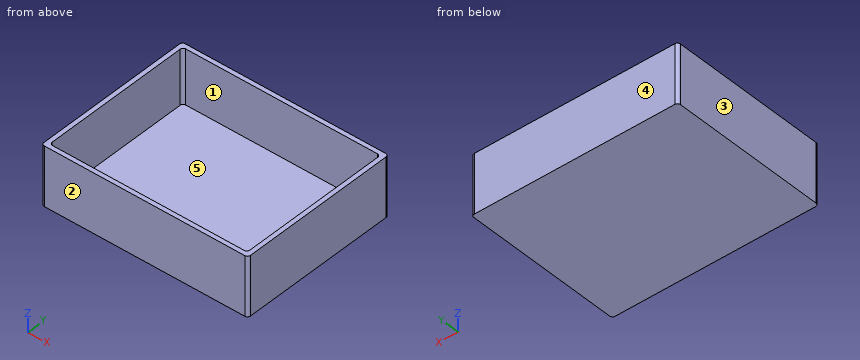
from build123d import *

# Parameters (mm, degrees)
F0_W     = 70
F0_H     = 55
F1_DEPTH = 20
F2_T     = -1.5
F3_R     = 1
F4_R     = 1
F5_R     = 1
F6_R     = 1
F7_R     = 1
F8_R     = 1
F9_R     = 1


with BuildPart() as f1:
    # F0 (on Top) → F1 (new body)
    with BuildSketch(Plane.XY):
        with Locations((35, 27.5)):
            Rectangle(F0_W, F0_H)
    extrude(amount=F1_DEPTH)

    # F2
    f2_openings = [f1.faces().sort_by_distance(p)[0] for p in [
        (35, 27.5, 20),
    ]]
    offset(amount=F2_T, openings=f2_openings)

    # F3
    f3_edges = [f1.edges().sort_by_distance(p)[0] for p in [
        (0, 55, 10),
        (1.5, 53.5, 10.75),
    ]]
    fillet(f3_edges, radius=F3_R)

    # F4
    f4_edges = [f1.edges().sort_by_distance(p)[0] for p in [
        (0, 0, 10),
    ]]
    fillet(f4_edges, radius=F4_R)

    # F5
    f5_edges = [f1.edges().sort_by_distance(p)[0] for p in [
        (70, 0, 10),
    ]]
    fillet(f5_edges, radius=F5_R)

    # F6
    f6_edges = [f1.edges().sort_by_distance(p)[0] for p in [
        (70, 55, 10),
    ]]
    fillet(f6_edges, radius=F6_R)

    # F7
    f7_edges = [f1.edges().sort_by_distance(p)[0] for p in [
        (68.5, 1.5, 10.75),
    ]]
    fillet(f7_edges, radius=F7_R)

    # F8
    f8_edges = [f1.edges().sort_by_distance(p)[0] for p in [
        (1.5, 1.5, 10.75),
    ]]
    fillet(f8_edges, radius=F8_R)

    # F9
    f9_edges = [f1.edges().sort_by_distance(p)[0] for p in [
        (68.5, 53.5, 10.75),
    ]]
    fillet(f9_edges, radius=F9_R)


solid = f1.part
Geometry: final body of the model. Coordinates: model frame, mm. Face numbers are marked on the shaded views. A direction names the side the tool comes from. Round coordinates to 2 decimals unless told otherwise and drop trailing zeros. Order: outer loops, then holes, each group sorted by start corner. A loop starts at its lowest first (then second) coordinate and runs counter-clockwise, first axis right, second up. Notation, with made-up numbers: (61, 26) -> (68, 26) arc R37 ccw to (68, 64) -> close; hole circle Ø2 at (49.25, 29.25). An arc over 180 degrees is marked (long way). Put each result on its own line as item: value. Start each with the question number.
Q1. Pull-direction query (Y, two-part tool) for the marked faces 1, 2 and 3; classes: +Y half, -Y half, draft (parallel to the pull), parting line (faces both ways), or undercut.
Q2. Reachability of the marked faces 4 and 5 from +Z, -Z, +X, -X, +Y, -Y: full face, straight path, thin tool, end or side. Return the list, or none.
Q3. Section A-A on x = 23. Return the cut outline in (y, z), and give its area (3 significant figures).
Q4. Section B-B on y = 6.5. Return the cut outline in (x, z).
Q5. First-contact query: pin 1 (4 mm diameter, centred on x = 13, y = 43.5, fed in from +Z). Flat tip, straight axial feed; report the tip coordinate or a pass-through.
Q6. Section C-C on z = 6. Return the cut outline in (x, y).
Q7. Line query: probe 1 along X at (y, z) = (33, 18.5); probe 2 along Y at (x, z) = (13, 10.5); probe 3 along Z at (x, y) = (26, 7). Output: solid intervals per line, ascending.
Ans:
1. face 1: undercut
1. face 2: -Y half
1. face 3: draft
2. face 4: +Z, -Z, +X, -X, +Y
2. face 5: +Z
3. outline: (0, 0) -> (55, 0) -> (55, 20) -> (53.5, 20) -> (53.5, 1.5) -> (1.5, 1.5) -> (1.5, 20) -> (0, 20) -> close
3. area: 138 mm2
4. outline: (0, 0) -> (70, 0) -> (70, 20) -> (68.5, 20) -> (68.5, 1.5) -> (1.5, 1.5) -> (1.5, 20) -> (0, 20) -> close
5. pin 1: stops at z = 1.5
6. outline: (0, 1) arc R1 ccw to (1, 0) -> (69, 0) arc R1 ccw to (70, 1) -> (70, 54) arc R1 ccw to (69, 55) -> (1, 55) arc R1 ccw to (0, 54) -> close; hole (1.5, 2.5) arc R1 ccw to (2.5, 1.5) -> (67.5, 1.5) arc R1 ccw to (68.5, 2.5) -> (68.5, 52.5) arc R1 ccw to (67.5, 53.5) -> (2.5, 53.5) arc R1 ccw to (1.5, 52.5) -> close
7. probe 1: x = 0 to 1.5, 68.5 to 70
7. probe 2: y = 0 to 1.5, 53.5 to 55
7. probe 3: z = 0 to 1.5
